Check sheet for the modelled part. Datum: model origin and axes. Units: mm. A direction names the side the tool comes from. Coordinates: 2 decimals unless noted, no trailing zeros. Write each loop counter-clockwise with the first axis right and the second up, starting at its lowest first coordinate (ties: lowest second). Pieces come first, ordered by that corner, then holes. Notation, with made-up numbers: (-21, -39) - (-2, -39) arc R21 ccw to (-2, -31) - close; hole circle Ø4 at (-33.75, 34.5). An arc over 180 degrees is marked (long way). Write each question's results on one line, items separated by ' | '.
from build123d import *

# Parameters (mm, degrees)
PAD_DEPTH            = 5
SKETCH017_W          = 56
SKETCH017_H          = 56
POCKET_DEPTH         = 5.001
POCKET_DEPTH_BACK    = 5.001
SKETCH004_R          = 2.5
POCKET010_DEPTH      = 69.501
POCKET010_DEPTH_BACK = 0.501
SKETCH003_R          = 2.5
POCKET011_DEPTH      = 0.001
POCKET011_DEPTH_BACK = 70.001


with BuildPart() as part:
    # Sketch → Pad (new body, symmetric)
    with BuildSketch(Plane.XY):
        with BuildLine():
            Line((-35, 32.113081), (-35, -32.113081))
            ThreePointArc((-35, -32.113081), (-33.587572, -33.587572), (-32.113081, -35))
            Line((-32.113081, -35), (32.113081, -35))
            ThreePointArc((32.113081, -35), (33.587572, -33.587572), (35, -32.113081))
            Line((35, -32.113081), (35, 32.113081))
            ThreePointArc((35, 32.113081), (33.587572, 33.587572), (32.113081, 35))
            Line((32.113081, 35), (-32.113081, 35))
            ThreePointArc((-32.113081, 35), (-33.587572, 33.587572), (-35, 32.113081))
        make_face()
    extrude(amount=PAD_DEPTH, both=True)

    # Sketch017 → Pocket (cut, two sides)
    with BuildSketch(Plane.XY) as pocket_sk:
        Rectangle(SKETCH017_W, SKETCH017_H)
    extrude(amount=-POCKET_DEPTH, mode=Mode.SUBTRACT)
    extrude(pocket_sk.sketch, amount=POCKET_DEPTH_BACK, mode=Mode.SUBTRACT)

    # Sketch004 → Pocket010 (cut, two sides)
    with BuildSketch(Plane(origin=(0, 34.5, 0), x_dir=(-1, 0, 0), z_dir=(0, 1, 0))) as pocket010_sk:
        Circle(SKETCH004_R)
    extrude(amount=-POCKET010_DEPTH, mode=Mode.SUBTRACT)
    extrude(pocket010_sk.sketch, amount=POCKET010_DEPTH_BACK, mode=Mode.SUBTRACT)

    # Sketch003 → Pocket011 (cut, two sides)
    with BuildSketch(Plane(origin=(-35, 0, 0), x_dir=(0, 0, -1), z_dir=(1, 0, 0))) as pocket011_sk:
        Circle(SKETCH003_R)
    extrude(amount=-POCKET011_DEPTH, mode=Mode.SUBTRACT)
    extrude(pocket011_sk.sketch, amount=POCKET011_DEPTH_BACK, mode=Mode.SUBTRACT)


solid = part.part
1. Sectioned sample at C-C (z = 0). Record the cut outline in (x, y).
Values follow:
outline: (-35, -32.11) arc R47.5 ccw to (-32.11, -35) - (-2.5, -35) - (-2.5, -28) - (-28, -28) - (-28, -2.5) - (-35, -2.5) - close; (-35, 2.5) - (-28, 2.5) - (-28, 28) - (-2.5, 28) - (-2.5, 35) - (-32.11, 35) arc R47.5 ccw to (-35, 32.11) - close; (2.5, -35) - (32.11, -35) arc R47.5 ccw to (35, -32.11) - (35, -2.5) - (28, -2.5) - (28, -28) - (2.5, -28) - close; (2.5, 28) - (28, 28) - (28, 2.5) - (35, 2.5) - (35, 32.11) arc R47.5 ccw to (32.11, 35) - (2.5, 35) - close
2. Sectioned sample at A-A (x = 10.5). Record the cut outline in (y, z), then the cut area to 3 significant figures.
Values follow:
outline: (-35, -5) - (-28, -5) - (-28, 5) - (-35, 5) - close; (28, -5) - (35, -5) - (35, 5) - (28, 5) - close | area: 140 mm^2
3. Sectioned sample at D-D (y = 0). Record the cut outline in (x, z).
Values follow:
outline: (-35, -5) - (-28, -5) - (-28, -2.5) - (-35, -2.5) - close; (-35, 2.5) - (-28, 2.5) - (-28, 5) - (-35, 5) - close; (28, -5) - (35, -5) - (35, -2.5) - (28, -2.5) - close; (28, 2.5) - (35, 2.5) - (35, 5) - (28, 5) - close
4. Go/stop test with a flat-tipped pin: pin 1 (4.5 mm diameter, centred on x = 0, z = 0, fed in from +Y). Record where the tip stops, or that it passes through.
Values follow:
pin 1: passes through
5. Draft check along Z on faces 1 (the flat face through (31, 0, 5)), 2 (the cylindrical face through (33.567, -33.608, 0.07)), 3 (the cylindrical face through (0.54, -31.45, -2.44)). Enter one of: pulls with the +Z half, pulls with the -Z half, needs draft (parallel to the pull), parting line crosses it, or undercut.
Values follow:
face 1: pulls with the +Z half | face 2: needs draft | face 3: undercut
6. Material ranges on L1, parallel to Z at x = 31, y = 0; L2, parallel to Y at x = 21, z = 1.75, recorded low to high. Write a range as [from, to].
Values follow:
L1: z = [-5, -2.5], [2.5, 5] | L2: y = [-35, -28], [28, 35]
7. Access from +Z, -Z, +X, -X, +Y, -Y to the whole of each face (thin tool, end or side, straight path). Record for faces 4 (the flat face through (-28, 0, 3)), 5 (the flat face through (-35, 0, 3)).
Values follow:
face 4: +Z, -Z | face 5: +Z, -Z, -X, +Y, -Y
